```python
from build123d import *

# Parameters (mm, degrees)
F0_W     = 25
F0_H     = 15
F1_DEPTH = 3.5
F2_R     = 1.65
F3_DEPTH = 3.5
F2_R_2   = 2.5
F4_DEPTH = 1


with BuildPart() as f1:
    # F0 (on Top) → F1 (new body)
    with BuildSketch(Plane.XY):
        Polygon((7.5, 20), (-7.5, 20), (-7.5, -20), (7.5, -20), (7.5, 5), align=None)
        with Locations((20, 12.5)):
            Rectangle(F0_W, F0_H)
    extrude(amount=F1_DEPTH)

    # F2 (on face) → F3 (cut, through all)
    with BuildSketch(Plane.XY.offset(3.5)):
        with Locations((0, 12.5)):
            Circle(F2_R)
        with Locations((0, -12)):
            Circle(F2_R)
        with Locations((24.5, 12.5)):
            Circle(F2_R)
    extrude(amount=-F3_DEPTH, mode=Mode.SUBTRACT)

    # F2 (on face) → F4 (cut)
    with BuildSketch(Plane.XY.offset(3.5)):
        with Locations((0, -12)):
            Circle(F2_R_2)
        with Locations((0, -12)):
            Circle(F2_R, mode=Mode.SUBTRACT)
        with Locations((0, 12.5)):
            Circle(F2_R_2)
        with Locations((0, 12.5)):
            Circle(F2_R, mode=Mode.SUBTRACT)
        with Locations((24.5, 12.5)):
            Circle(F2_R_2)
        with Locations((24.5, 12.5)):
            Circle(F2_R, mode=Mode.SUBTRACT)
    extrude(amount=-F4_DEPTH, mode=Mode.SUBTRACT)


solid = f1.part
```
The model under review builds one solid part; all positions refer to its coordinate system, in mm. A direction names the side the tool comes from. Round coordinates to 2 decimals unless told otherwise and drop trailing zeros. Loops run counter-clockwise (first coordinate to the right, second up) from the corner with the lowest first, then second, coordinate; pieces in that order, holes last. Notation, with made-up numbers: M -25,-19.75 L 0,-19.75 A13 ccw 0,-2.75 Z; hole C -32,-12.75 d4. An arc over 180 degrees is marked long. Answer as a JSON object with one key per item and string values.
(1) Take a section at D-D on z = 2. Give the boundary of the cut face in (x, y), and give its area (3 significant figures).
Resolved:
{"outline": "M -7.5,-20 L 7.5,-20 L 7.5,5 L 32.5,5 L 32.5,20 L -7.5,20 Z; hole C 0,-12 d3.3; hole C 0,12.5 d3.3; hole C 24.5,12.5 d3.3", "area": "949 mm²"}
(2) Take a section at C-C on x = 0. Give the boundary of the cut face in (y, z).
Resolved:
{"outline": "M -20,0 L -13.65,0 L -13.65,2.5 L -14.5,2.5 L -14.5,3.5 L -20,3.5 Z; M -10.35,0 L 10.85,0 L 10.85,2.5 L 10,2.5 L 10,3.5 L -9.5,3.5 L -9.5,2.5 L -10.35,2.5 Z; M 14.15,0 L 20,0 L 20,3.5 L 15,3.5 L 15,2.5 L 14.15,2.5 Z"}
(3) Draft analysis for pull direction Y (two halves, no side actions). For faces 4 (the flat face through (-7.5, 0, 2)), 5 (the flat face through (0, -20, 2)), 6 (the cylindrical face through (-0.54, -14.44, 3.01)), state which applies: released by +Y, released by -Y, zero draft, split by the parting line, or undercut.
Resolved:
{"face 4": "zero draft", "face 5": "released by -Y", "face 6": "undercut"}
(4) Tool access review of faces 1 (the cylindrical face through (-0.4, 10.9, 1.3)), 2 (the cylindrical face through (-0.54, 10.06, 3.01)), 3 (the flat face through (7.5, -8, 2)): name each direction out of +Z, -Z, +X, -X, +Y, -Y from which nothing blocks a thin tool from reaching the whole face with its end or side.
Resolved:
{"face 1": "+Z, -Z", "face 2": "+Z", "face 3": "+Z, -Z, +X, -Y"}
(5) Take a section at B-B on y = 12.5. Give the boundary of the cut face in (x, z), and give its area (4 significant figures).
Resolved:
{"outline": "M -7.5,0 L -1.65,0 L -1.65,2.5 L -2.5,2.5 L -2.5,3.5 L -7.5,3.5 Z; M 1.65,0 L 22.85,0 L 22.85,2.5 L 22,2.5 L 22,3.5 L 2.5,3.5 L 2.5,2.5 L 1.65,2.5 Z; M 26.15,0 L 32.5,0 L 32.5,3.5 L 27,3.5 L 27,2.5 L 26.15,2.5 Z", "area": "113.5 mm²"}
(6) Take a section at A-A on x = 24.5. Give the boundary of the cut face in (y, z).
Resolved:
{"outline": "M 5,0 L 10.85,0 L 10.85,2.5 L 10,2.5 L 10,3.5 L 5,3.5 Z; M 14.15,0 L 20,0 L 20,3.5 L 15,3.5 L 15,2.5 L 14.15,2.5 Z"}
(7) To check wall thickness, follow line 1 along Y through (x, z) = (24.5, 1.5); line 2 along Y through (x, z) = (0, 1.25); line 3 along Y through (x, z) = (19, 1.25). State the ranges of each line that lie inside material, in increasing order.
Resolved:
{"line 1": "5 to 10.85, 14.15 to 20", "line 2": "-20 to -13.65, -10.35 to 10.85, 14.15 to 20", "line 3": "5 to 20"}
(8) Clearance check with flat-ended pins moving along their axes: P1, Ø1.5, axis at x = 1, y = 13, coming from the +Z side; P2, Ø1.8, axis at x = 20.5, z = 1, coming from the -Y side. State where each tip first meets the part, or that it passes through.
Resolved:
{"P1": "z = 2.5", "P2": "y = 5"}
